Can you work these out from the model? Positions are in its coordinate system, mm. A direction names the side the tool comes from. Round coordinates to 2 decimals unless told otherwise and drop trailing zeros. Order: outer loops, then holes, each group sorted by start corner. A loop starts at its lowest first (then second) coordinate and runs counter-clockwise, first axis right, second up.
Q1. If I drill on line 1 (Z direction, x = 11, y = 14); line 2 (Y direction, x = 18.5, z = 29); line 3 (X direction, y = -6, z = 60.5) (3 decimals), over which ranges is the centre line in solid material (lowest first)?
Q2. If we section it at A-A (y = 4.5): Please give me the cut outline in (x, z), plus the area to 3 significant figures.
Q3. If we section it at C-C (z = 34.5): Please give me the cut outline in (x, y), plus the area to 3 significant figures.
Q4. If we section it at D-D (y = 17.5): Please give me the cut outline in (x, z), plus the area to 3 significant figures.
Q5. For faces 1 (the face through (25, 0, 40)), 2 (the face through (0, -7.5, 53)), 3 (the face through (0, 7.5, 53)), 4 (the face through (-25, 0, 40)), which set-ups out of +Z, -Z, +X, -X, +Y, -Y let a thin tool reach every point of the face, with its end or its side?
Q6. Will these pins go through, and if not, where does the flat tip stop? P1, Ø6, axis at x = 3, y = -16.5, coming from the +Z side; P2, Ø6, axis at y = -3.5, z = 66, coming from the -X side; P3, Ø8, axis at y = 2.5, z = 28.5, coming from the +X side.
Q7. If we section it at B-B (x = 0): Please give me the cut outline in (y, z).
from build123d import *

# Parameters (mm, degrees)
F0_W     = 100
F0_H     = 50
F1_DEPTH = 20
F2_SIZE  = 8
F4_DEPTH = 7.5


with BuildPart() as f1:
    # F0 (on Top) → F1 (new body)
    with BuildSketch(Plane.XY):
        Rectangle(F0_W, F0_H)
    extrude(amount=F1_DEPTH)

    # F2
    f2_edges = [f1.edges().sort_by_distance(p)[0] for p in [
        (-50, 0, 20),
        (50, 0, 20),
    ]]
    chamfer(f2_edges, length=F2_SIZE)

    # F3 (on Front) → F4 (join, symmetric)
    with BuildSketch(Plane.XZ):
        with BuildLine():
            Line((-25, 60), (-25, 20))
            Line((-25, 20), (25, 20))
            Line((25, 20), (25, 60))
            ThreePointArc((25, 60), (0, 85), (-25, 60))
        make_face()
    extrude(amount=F4_DEPTH, both=True)


solid = f1.part
Solution:
1. line 1: z = 0 to 20
1. line 2: y = -7.5 to 7.5
1. line 3: x = -24.995 to 24.995
2. outline: (-50, 0) - (50, 0) - (50, 12) - (42, 20) - (25, 20) - (25, 60) arc R25 ccw to (-25, 60) - (-25, 20) - (-42, 20) - (-50, 12) - close
2. area: 4,920 mm2
3. outline: (-25, -7.5) - (25, -7.5) - (25, 7.5) - (-25, 7.5) - close
3. area: 750 mm2
4. outline: (-50, 0) - (50, 0) - (50, 12) - (42, 20) - (-42, 20) - (-50, 12) - close
4. area: 1,940 mm2
5. face 1: +Z, +X, +Y, -Y
5. face 2: +Z, +X, -X, -Y
5. face 3: +Z, +X, -X, +Y
5. face 4: +Z, -X, +Y, -Y
6. P1: stops at z = 20
6. P2: stops at x = -24.82
6. P3: stops at x = 25
7. outline: (-25, 0) - (25, 0) - (25, 20) - (7.5, 20) - (7.5, 85) - (-7.5, 85) - (-7.5, 20) - (-25, 20) - close
